```python
from build123d import *

# Parameters (mm, degrees)
F0_W     = 137.842797
F0_H     = 77.237847
F1_DEPTH = 60
F2_R     = 16.906171
F3_DEPTH = 25
F4_R     = 5


with BuildPart() as f1:
    # F0 (on Top) → F1 (new body)
    with BuildSketch(Plane.XY):
        with Locations((0.66914, 8.698817)):
            Rectangle(F0_W, F0_H)
    extrude(amount=F1_DEPTH)

    # F2 (on face) → F3 (cut)
    with BuildSketch(Plane.XY.offset(60)):
        with Locations((45.942705, -4.954772)):
            Circle(F2_R)
    extrude(amount=-F3_DEPTH, mode=Mode.SUBTRACT)

    # F4
    f4_edges = [f1.edges().sort_by_distance(p)[0] for p in [
        (0.66914, -29.920107, 60),
        (69.590539, 8.698816, 60),
        (0.66914, 47.31774, 60),
        (-68.252258, 8.698816, 60),
    ]]
    fillet(f4_edges, radius=F4_R)


solid = f1.part
```
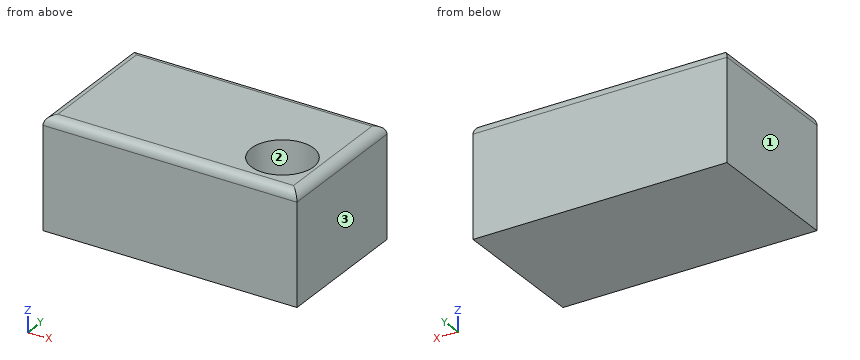
Work out the finished part from the listing and answer in its coordinate system (mm). Face numbers are marked on the shaded views. Coordinates: 2 decimals unless noted, no trailing zeros. Write each loop counter-clockwise with the first axis right and the second up, starting at its lowest first coordinate (ties: lowest second). Pieces come first, ordered by that corner, then holes. Notation, with made-up numbers: (-32.75, -30) - (17.25, -30) arc R26 cw to (17.25, -9) - close; hole circle Ø7 at (36, 86). An arc over 180 degrees is marked (long way). Answer as a JSON object with one key per item and string values.
Q1. Given pin 1 Ø4 at (x, y) = (50, -4.5) entering from +Z, flat-ended and moving along its own axis, determine where the tip first touches the part or whether it passes through.
Results list:
{"pin 1": "stops at z = 35"}
Q2. Find section A-A (x = 37.5). Write down the section's boundary in (y, z), plus the area to 3 significant figures.
Results list:
{"outline": "(-29.92, 0) - (47.32, 0) - (47.32, 55) arc R5 ccw to (42.32, 60) - (9.69, 60) - (9.69, 35) - (-19.6, 35) - (-19.6, 60) - (-24.92, 60) arc R5 ccw to (-29.92, 55) - close", "area": "3,890 mm^2"}
Q3. For a pull along X with two mould halves and no side action, classify the marked faces 1, 2 and 3 as pulls with the +X half, pulls with the -X half, needs draft (parallel to the pull), parting line crosses it, or undercut.
Results list:
{"face 1": "pulls with the -X half", "face 2": "undercut", "face 3": "pulls with the +X half"}
Q4. Consider L1, parallel to Y at x = 39.5, z = 48.5; L2, parallel to Z at x = 55.5, y = -9.5; L3, parallel to X at y = -17.5, z = 50. Determine where each line is inside the solid, lowest interval first. Write a range as from..to.
Results list:
{"L1": "y = -29.92..-20.59, 10.68..47.32", "L2": "z = 0..35", "L3": "x = -68.25..34.61, 57.28..69.59"}
Q5. Find section B-B (y = -3). Write down the section's boundary in (x, z), plus the area to 3 significant figures.
Results list:
{"outline": "(-68.25, 0) - (69.59, 0) - (69.59, 55) arc R5 ccw to (64.59, 60) - (62.74, 60) - (62.74, 35) - (29.15, 35) - (29.15, 60) - (-63.25, 60) arc R5 ccw to (-68.25, 55) - close", "area": "7,420 mm^2"}
Q6. Find section C-C (z = 41.5). Write down the section's boundary in (x, y), plus the area to 3 significant figures.
Results list:
{"outline": "(-68.25, -29.92) - (69.59, -29.92) - (69.59, 47.32) - (-68.25, 47.32) - close; hole circle Ø33.81 at (45.94, -4.95)", "area": "9,750 mm^2"}
